Answer from the drawing. Dimensions are ordinates in mm from the lowest x, y and z of the part. A direction names the side the tool comes from. Give positions to 0.01 mm unless a question says otherwise; leave off trailing zeros. Loops run counter-clockwise (first coordinate to the right, second up) from the corner with the lowest first, then second, coordinate; pieces in that order, holes last. Notation, with made-up numbers: (29.5, 29) - (64.5, 29) arc R26 cw to (64.5, 59) - close; hole circle Ø5 at (36.5, 17.5). An arc over 180 degrees is marked (long way). One line per item, written item: value.
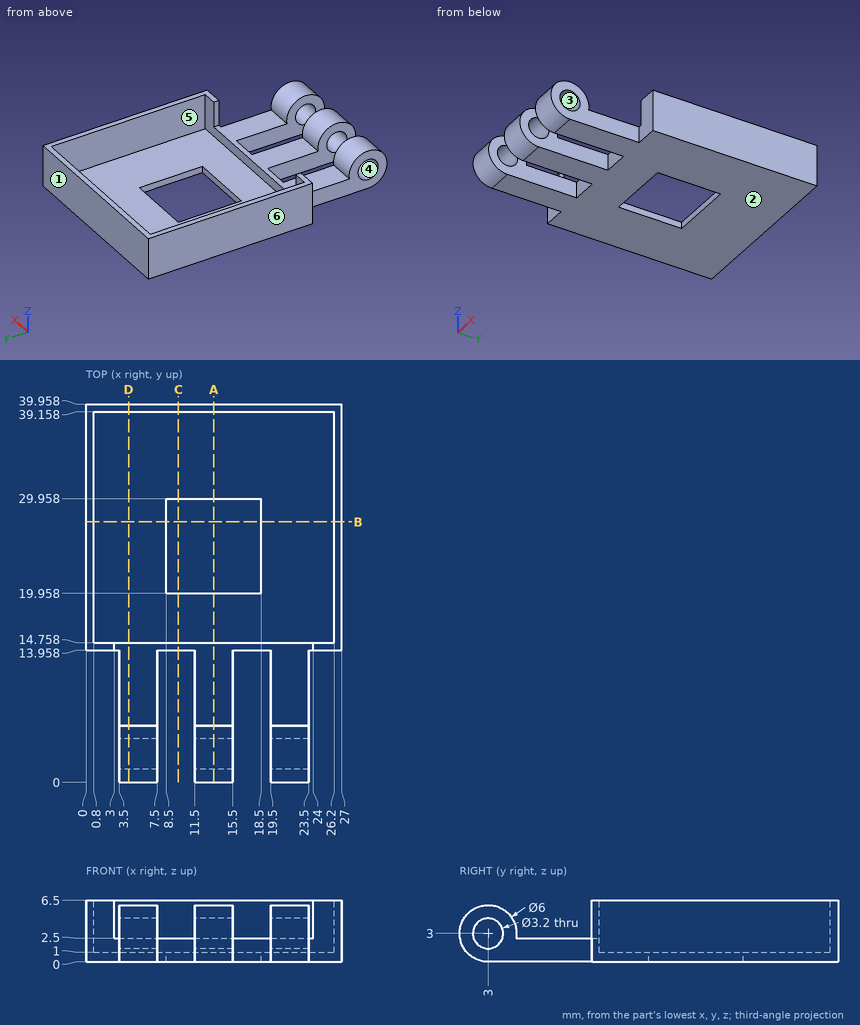
1. Section B-B (y = 27.5) is taken. Write down the section's boundary in (x, z).
Output:
outline: (0, 0) - (8.5, 0) - (8.5, 1) - (0.8, 1) - (0.8, 6.5) - (0, 6.5) - close; (18.5, 0) - (27, 0) - (27, 6.5) - (26.2, 6.5) - (26.2, 1) - (18.5, 1) - close
2. The mould has two halves that part along Z. Classify the marked faces 1, 2, 3 and 4: released by +Z, released by -Z, zero draft, split by the parting line, or undercut.
Output:
face 1: zero draft
face 2: released by -Z
face 3: undercut
face 4: undercut
3. Section C-C (x = 9.75) is taken. Write down the section's boundary in (y, z), and give its area (3 significant figures).
Output:
outline: (13.96, 0) - (19.96, 0) - (19.96, 1) - (14.76, 1) - (14.76, 2.5) - (13.96, 2.5) - close; (29.96, 0) - (39.96, 0) - (39.96, 6.5) - (39.16, 6.5) - (39.16, 1) - (29.96, 1) - close
area: 21.6 mm²
4. Section D-D (x = 4.5) is taken. Write down the section's boundary in (y, z).
Output:
outline: (3, 0) - (39.96, 0) - (39.96, 6.5) - (39.16, 6.5) - (39.16, 1) - (14.76, 1) - (14.76, 2.5) - (5.96, 2.5) arc R3 ccw (long way) to start; hole circle Ø3.2 at (3, 3)
5. For the marked faces 5 and 6, determine the directions among +Z, -Z, +X, -X, +Y, -Y from which every point of the face is accessible in a straight line to the end or side of a thin tool.
Output:
face 5: +Z
face 6: +Z, -Z, -X, +Y, -Y
6. Flat-ended cylindrical pins translate along their axes: pin 1 Ø1.8 at (y, z) = (9, 4) entering from -X; pin 2 Ø1 at (x, z) = (21, 5) entering from -Y; pin 3 Ø1.5 at (x, z) = (22, 0.5) entering from -Y; pin 4 Ø3.5 at (y, z) = (3, 3) entering from -X. Find the tip coordinate at first contact, or state that the pin passes through.
Output:
pin 1: passes through
pin 2: stops at y = 0.4
pin 3: stops at y = 0.56
pin 4: stops at x = 3.5
7. Section A-A (x = 13.5) is taken. Write down the section's boundary in (y, z).
Output:
outline: (3, 0) - (19.96, 0) - (19.96, 1) - (14.76, 1) - (14.76, 2.5) - (5.96, 2.5) arc R3 ccw (long way) to start; (29.96, 0) - (39.96, 0) - (39.96, 6.5) - (39.16, 6.5) - (39.16, 1) - (29.96, 1) - close; hole circle Ø3.2 at (3, 3)
8. Find the intervals of material crossed by line 1 along Y through (x, z) = (6.3, 3); line 2 along Y through (x, z) = (24, 1.25); line 3 along X through (y, z) = (29.5, 6), in increasing order.
Output:
line 1: y = 0 to 1.4, 4.6 to 6, 39.16 to 39.96
line 2: y = 13.96 to 14.76, 39.16 to 39.96
line 3: x = 0 to 0.8, 26.2 to 27
